Part model, mm, in its own coordinate system. Face numbers are marked on the shaded views. A direction names the side the tool comes from. Give positions to 0.01 mm unless a question says otherwise; leave off trailing zeros. Order: outer loops, then holes, each group sorted by start corner. A loop starts at its lowest first (then second) coordinate and runs counter-clockwise, first axis right, second up. Notation, with made-up numbers: (33, 75) - (41, 75) arc R19 ccw to (41, 86) - close; hole circle Ø4 at (18.5, 55.5). An arc over 180 degrees is marked (long way). One line per item, written item: value.
```python
from build123d import *

# Parameters (mm, degrees)
BOSS_EXTRUDE1_DEPTH   = 12.5
F_4_CLEARANCE_HOLE1_D = 3.2639
F_1_CLEARANCE_HOLE1_D = 2.0574
SKETCH7_W             = 12.7
SKETCH7_H             = 28
CUT_EXTRUDE1_DEPTH    = 4.4


with BuildPart() as part:
    # Sketch1 → Boss-Extrude1 (new, symmetric)
    with BuildSketch(Plane.XY):
        Polygon((15, 0), (0, 0), (0, 35), (1.5875, 35), (1.5875, 1.5875), (15, 1.5875), align=None)
    extrude(amount=BOSS_EXTRUDE1_DEPTH, both=True)

    # #4 Clearance Hole1 (through all)
    with Locations(Plane(origin=(0, 0, 0), x_dir=(-1, 0, 0), z_dir=(0, -1, 0))):
        with Locations((-7.5, 10), (-7.5, -10)):
            Hole(F_4_CLEARANCE_HOLE1_D / 2)

    # #1 Clearance Hole1 (through all)
    with Locations(Plane.ZY):
        with Locations((0, 30.19)):
            Hole(F_1_CLEARANCE_HOLE1_D / 2)

    # Sketch7 → Cut-Extrude1 (cut)
    with BuildSketch(Plane.ZY):
        with Locations((0, 14)):
            Rectangle(SKETCH7_W, SKETCH7_H)
    extrude(amount=-CUT_EXTRUDE1_DEPTH, mode=Mode.SUBTRACT)


solid = part.part
```
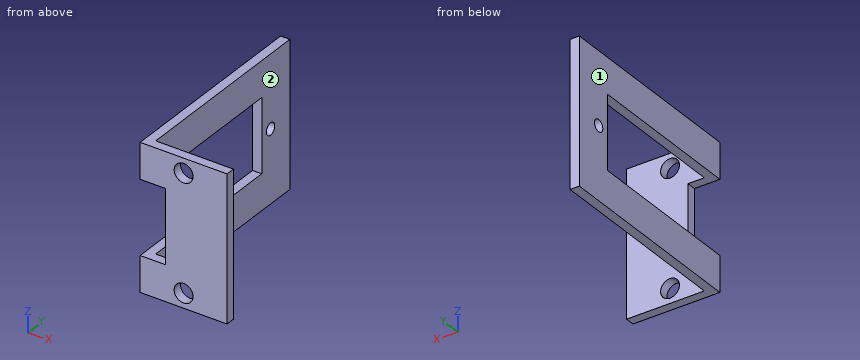
1) Cut at C-C, the plane x = 7.5. Give the cut face in (y, z).
Outcome:
outline: (0, -12.5) - (1.59, -12.5) - (1.59, -11.63) - (0, -11.63) - close; (0, -8.37) - (1.59, -8.37) - (1.59, 8.37) - (0, 8.37) - close; (0, 11.63) - (1.59, 11.63) - (1.59, 12.5) - (0, 12.5) - close
2) Cut at D-D, the plane z = 10. Give the cut face in (x, y), then the cut area to 3 significant figures.
Outcome:
outline: (0, 0) - (5.87, 0) - (5.87, 1.59) - (1.59, 1.59) - (1.59, 35) - (0, 35) - close; (9.13, 0) - (15, 0) - (15, 1.59) - (9.13, 1.59) - close
area: 71.7 mm^2
3) Which spindle directions (+Z, -Z, +X, -X, +Y, -Y) get a long thin tool onto all of the face, cutting with end or side? Do the marked faces 1 and 2. Say none if no direction does.
Outcome:
face 1: +Z, -Z, -X, +Y, -Y
face 2: +Z, -Z, +X, +Y
4) Drill centre lines: line 1 along Z through (x, y) = (7.5, 0.4); line 2 along X through (y, z) = (1, -10); line 3 along Y through (x, z) = (0.75, 0). Where is each one in solid material? Low to high. Write a range as from..to.
Outcome:
line 1: z = -12.5..-11.63, -8.37..8.37, 11.63..12.5
line 2: x = 0..5.87, 9.13..15
line 3: y = 28..29.16, 31.22..35
5) Cut at A-A, the plane y = 30.19. Give the cut face in (x, z).
Outcome:
outline: (0, -12.5) - (1.59, -12.5) - (1.59, -1.03) - (0, -1.03) - close; (0, 1.03) - (1.59, 1.03) - (1.59, 12.5) - (0, 12.5) - close
6) Pin check, flat tips, straight feed: pin 1 (5 mm diameter, centred on x = 13, z = 4, fed in from +Y); pin 2 (7.5 mm diameter, centred on y = 25, z = -2.5, fed in from +X); pin 3 (1.2 mm diameter, centred on y = 30.19, z = 0, fed in from -X); pin 4 (1.3 mm diameter, centred on y = 1, z = 1, fed in from -X). Stop position of each tip, or through.
Outcome:
pin 1: stops at y = 1.59
pin 2: stops at x = 1.59
pin 3: passes through
pin 4: stops at x = 4.4
7) Cut at B-B, the plane z = 0. Give the cut face in (x, y), then the cut area to 3 significant figures.
Outcome:
outline: (0, 28) - (1.59, 28) - (1.59, 29.16) - (0, 29.16) - close; (0, 31.22) - (1.59, 31.22) - (1.59, 35) - (0, 35) - close; (4.4, 0) - (15, 0) - (15, 1.59) - (4.4, 1.59) - close
area: 24.7 mm^2
